```python
from build123d import *

# Parameters (mm, degrees)
SKIZZE1_R                       = 10
AUFSATZ_LINEAR_AUSTRAGEN1_DEPTH = 204
SKIZZE2_R                       = 10
SKIZZE2_R_2                     = 8
SCHNITT_LINEAR_AUSTRAGEN1_DEPTH = 31
SKIZZE3_R                       = 10
SKIZZE3_R_2                     = 8
SCHNITT_LINEAR_AUSTRAGEN2_DEPTH = 28
FASE1_SIZE                      = 2
FASE2_SIZE                      = 2


with BuildPart() as part:
    # Skizze1 → Aufsatz-Linear austragen1 (new body)
    with BuildSketch(Plane.XY):
        Circle(SKIZZE1_R)
    extrude(amount=AUFSATZ_LINEAR_AUSTRAGEN1_DEPTH)

    # Skizze2 → Schnitt-Linear austragen1 (cut)
    with BuildSketch(Plane(origin=(0, 0, 0), x_dir=(-1, 0, 0), z_dir=(0, 0, -1))):
        Circle(SKIZZE2_R)
        Circle(SKIZZE2_R_2, mode=Mode.SUBTRACT)
    extrude(amount=-SCHNITT_LINEAR_AUSTRAGEN1_DEPTH, mode=Mode.SUBTRACT)

    # Skizze3 → Schnitt-Linear austragen2 (cut)
    with BuildSketch(Plane.XY.offset(204)):
        Circle(SKIZZE3_R)
        Circle(SKIZZE3_R_2, mode=Mode.SUBTRACT)
    extrude(amount=-SCHNITT_LINEAR_AUSTRAGEN2_DEPTH, mode=Mode.SUBTRACT)

    # Fase1
    fase1_edges = [part.edges().sort_by_distance(p)[0] for p in [
        (-8, 0, 204),
    ]]
    chamfer(fase1_edges, length=FASE1_SIZE)

    # Fase2
    fase2_edges = [part.edges().sort_by_distance(p)[0] for p in [
        (8, 0, 0),
    ]]
    chamfer(fase2_edges, length=FASE2_SIZE)


solid = part.part
```
The model under review builds one solid part; all positions refer to its coordinate system, in mm. A direction names the side the tool comes from. Round coordinates to 2 decimals unless told otherwise and drop trailing zeros. Order: outer loops, then holes, each group sorted by start corner. A loop starts at its lowest first (then second) coordinate and runs counter-clockwise, first axis right, second up.
Item 1: Add section A-A, the plane y = 0. State the section outline as (x, z) points.
Working result:
outline: (-10, 31) - (-8, 31) - (-8, 2) - (-6, 0) - (6, 0) - (8, 2) - (8, 31) - (10, 31) - (10, 176) - (8, 176) - (8, 202) - (6, 204) - (-6, 204) - (-8, 202) - (-8, 176) - (-10, 176) - close
Item 2: Add section C-C, the plane z = 49.5. State the section outline as (x, y) points, and give its area (3 significant figures).
Working result:
outline: circle Ø20 at (0, 0)
area: 314 mm2
Item 3: For pin 1 (8 mm diameter, centred on x = 7, z = 65.5, fed in from -Y); pin 2 (3 mm diameter, centred on y = -3, z = 49, fed in from -X); pin 3 (4 mm diameter, centred on x = 7, y = -6, fed in from +Z), all flat-tipped, find the tip position at first contact; note any pin that passes through.
Working result:
pin 1: stops at y = -9.54
pin 2: stops at x = -9.89
pin 3: stops at z = 202.78
Item 4: To check wall thickness, follow probe 1 along Z at (x, y) = (-7.5, -5.5); probe 2 along Y at (x, z) = (-8, 62); probe 3 along X at (y, z) = (-6, 32). State the ranges of each line that lie inside material, in increasing order.
Working result:
probe 1: z = 31 to 176
probe 2: y = -6 to 6
probe 3: x = -8 to 8
Item 5: Machinability: for faces 1 (the flat face through (0, 8.2, 176)), 2 (the cylindrical face through (1.73, -7.81, 16.3)), 3 (the flat face through (0, 0, 204)), which of the approach directions +Z, -Z, +X, -X, +Y, -Y give a long, thin tool a straight path to every point of the face, cutting with its end or side? Answer none if there is none.
Working result:
face 1: +Z
face 2: -Z
face 3: +Z, +X, -X, +Y, -Y
